Geometry check sheet. Reference: drawing and pictorial views, mm from the part's lowest x, y, z. Coordinates: 2 decimals unless noted, no trailing zeros. Write each loop counter-clockwise with the first axis right and the second up, starting at its lowest first coordinate (ties: lowest second). Pieces come first, ordered by that corner, then holes. Notation, with made-up numbers: (6.25, 46.25) -> (23.25, 46.25) arc R30 ccw to (23.25, 80.25) -> close; hole circle Ø9 at (61.5, -6.5). An arc over 180 degrees is marked (long way). Answer in a Markdown table with one row per item.
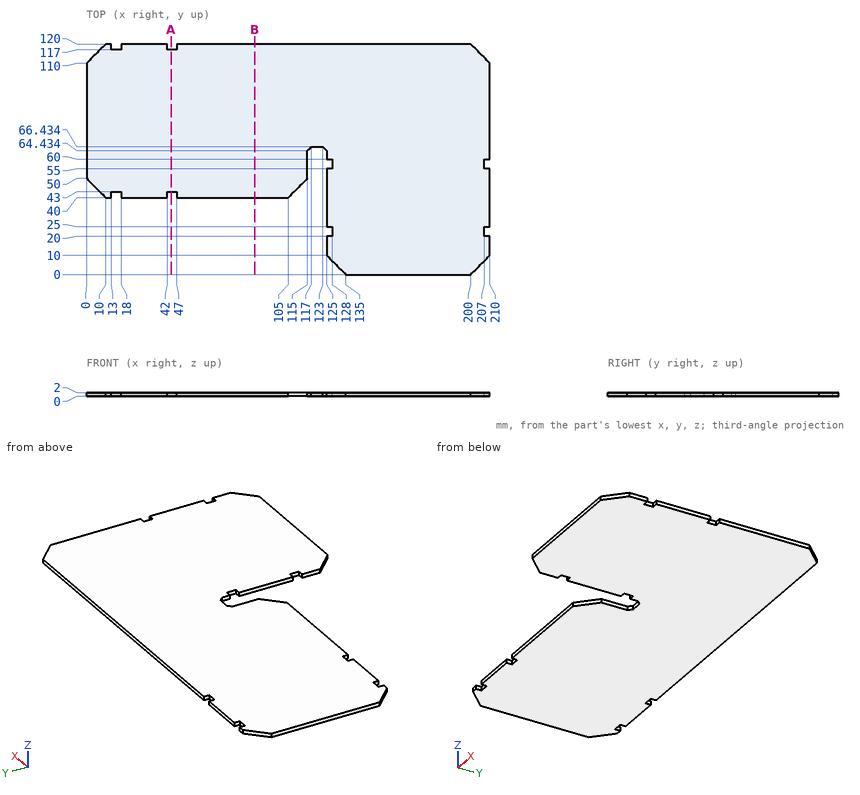
1. Section check B-B, the plane x = 87.5. Record the boundary of the cut face in (y, z).
Geometry says:
| item | result |
|---|---|
| outline | (40, 0) -> (120, 0) -> (120, 2) -> (40, 2) -> close |
2. Thickness scan on line 1 (X direction, y = 55.5, z = 0.5); line 2 (X direction, y = 53, z = 0.35); line 3 (X direction, y = 15, z = 0.25). Record the ranges inside material, lowest first. Write a range as from..to.
Geometry says:
| item | result |
|---|---|
| line 1 | 0..115, 128..207 |
| line 2 | 0..115, 125..210 |
| line 3 | 125..210 |
3. Depth check by flat-ended pin: P1, Ø8, axis at x = 137.5, y = 102, coming from the -Z side; P2, Ø0.6, axis at x = 208.5, z = 1, coming from the -Y side; P3, Ø0.6, axis at y = 39.5, z = 1.5, coming from the -X side; P4, Ø1, axis at x = 121, z = 1, coming from the -Y side. Enter the tip coordinate at first touch or a pass-through.
Geometry says:
| item | result |
|---|---|
| P1 | z = 0 |
| P2 | y = 8.2 |
| P3 | x = 125 |
| P4 | y = 66.43 |
4. Section check A-A, the plane x = 44. Record the boundary of the cut face in (y, z).
Geometry says:
| item | result |
|---|---|
| outline | (43, 0) -> (117, 0) -> (117, 2) -> (43, 2) -> close |
